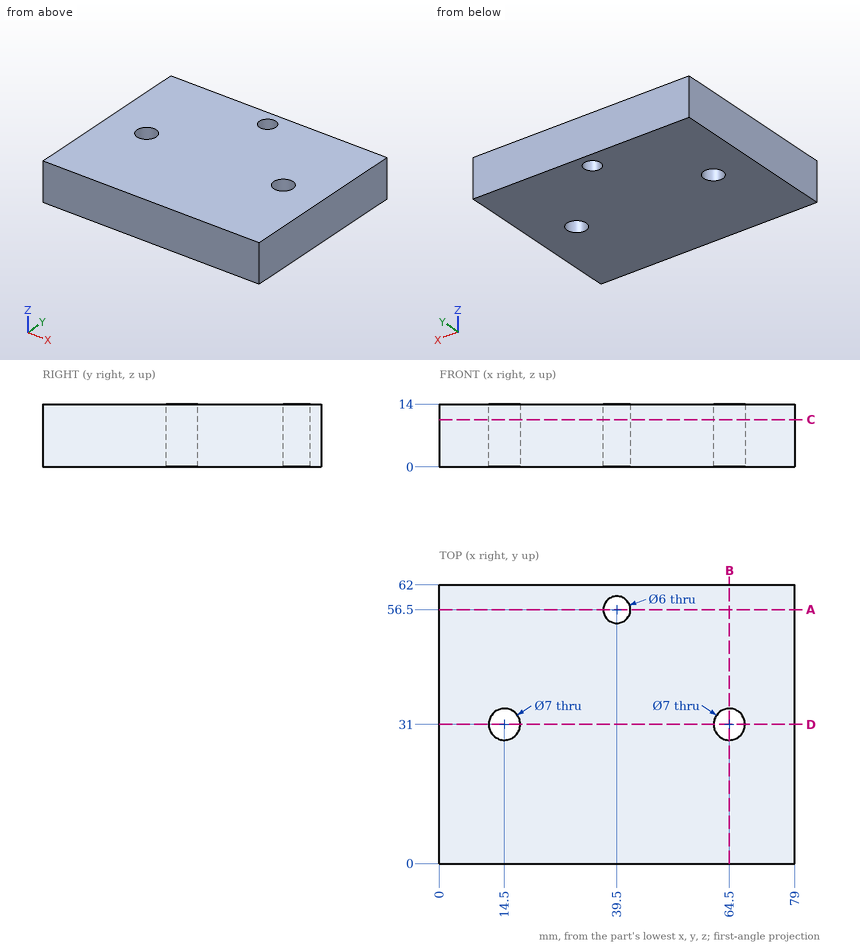
Geometry check sheet. Reference: drawing and pictorial views, mm from the part's lowest x, y, z. Round coordinates to 2 decimals unless told otherwise and drop trailing zeros. Order: outer loops, then holes, each group sorted by start corner. A loop starts at its lowest first (then second) coordinate and runs counter-clockwise, first axis right, second up. Notation, with made-up numbers: M -7.5,34 L 23.5,34 A22 ccw 23.5,49 Z; hole C 47,75.25 d9. An arc over 180 degrees is marked long. Write item = value, one per line.
Q1. Section check A-A (y = 56.5). Enter the section's corners in (x, z), plus the area to 3 significant figures.
Answer block:
outline = M 0,0 L 36.5,0 L 36.5,14 L 0,14 Z; M 42.5,0 L 79,0 L 79,14 L 42.5,14 Z
area = 1,020 mm^2
Q2. Section check B-B (x = 64.5). Enter the section's corners in (y, z).
Answer block:
outline = M 0,0 L 27.5,0 L 27.5,14 L 0,14 Z; M 34.5,0 L 62,0 L 62,14 L 34.5,14 Z
Q3. Depth check by flat-ended pin: pin 1 Ø11 at (x, y) = (64.5, 31) entering from -Z. Enter the tip coordinate at first touch or a pass-through.
Answer block:
pin_1 = 0
Q4. Scan lines: line 1 (Y direction, x = 14.5, z = 4.5); line 2 (Y direction, x = 39.5, z = 5.25); line 3 (X direction, y = 56, z = 6). Record each from-to range of solid material in increasing order.
Answer block:
line_1 = 0 to 27.5, 34.5 to 62
line_2 = 0 to 53.5, 59.5 to 62
line_3 = 0 to 36.54, 42.46 to 79
Q5. Section check D-D (y = 31). Enter the section's corners in (x, z), plus the area to 3 significant figures.
Answer block:
outline = M 0,0 L 11,0 L 11,14 L 0,14 Z; M 18,0 L 61,0 L 61,14 L 18,14 Z; M 68,0 L 79,0 L 79,14 L 68,14 Z
area = 910 mm^2
Q6. Section check C-C (z = 10.5). Enter the section's corners in (x, y).
Answer block:
outline = M 0,0 L 79,0 L 79,62 L 0,62 Z; hole C 14.5,31 d7; hole C 39.5,56.5 d6; hole C 64.5,31 d7
